Could you check a few things on this model? Use its own coordinates, in mm. Face numbers are marked on the shaded views. A direction names the side the tool comes from. Coordinates: 2 decimals unless noted, no trailing zeros. Write each loop counter-clockwise with the first axis right and the second up, starting at its lowest first coordinate (ties: lowest second). Pieces come first, ordered by that corner, then holes.
```python
from build123d import *

# Parameters (mm, degrees)
CROQUIS1_R              = 1.5
SALIENTE_EXTRUIR1_DEPTH = 10
CROQUIS2_R              = 1.5
CORTAR_EXTRUIR1_DEPTH   = 10
CROQUIS3_W              = 30
CROQUIS3_H              = 5.454139521
CORTAR_EXTRUIR2_DEPTH   = 10
REDONDEO1_R             = 5
CORTAR_EXTRUIR3_DEPTH   = 10


with BuildPart() as part:
    # Croquis1 → Saliente-Extruir1 (new body)
    with BuildSketch(Plane.XY):
        Polygon((0, 0), (15, 0), (15, 2.5), (25, 2.5), (25, 7.5), (15, 7.5), (15, 10), (0, 10), align=None)
        with Locations((5, 5)):
            Circle(CROQUIS1_R, mode=Mode.SUBTRACT)
    extrude(amount=SALIENTE_EXTRUIR1_DEPTH)

    # Croquis2 → Cortar-Extruir1 (cut)
    with BuildSketch(Plane(origin=(0, 7.5, 0), x_dir=(1, 0, 0), z_dir=(0, 1, 0))):
        with Locations(Location((20, -5, 0), (0, 0, 270))):
            Circle(CROQUIS2_R)
        with BuildLine():
            Line((20, -10), (20.922664414, -18.434540281))
            Line((20.922664414, -18.434540281), (42.481308924, -25.135304993))
            Line((42.481308924, -25.135304993), (36.797179784, -0.604681732))
            Line((36.797179784, -0.604681732), (34.226694382, 7.989532519))
            Line((34.226694382, 7.989532519), (20.461332207, 6.483723144))
            Line((20.461332207, 6.483723144), (20, 0))
            ThreePointArc((20, 0), (25, -5), (20, -10))
        make_face()
    extrude(amount=-CORTAR_EXTRUIR1_DEPTH, mode=Mode.SUBTRACT)

    # Croquis3 → Cortar-Extruir2 (cut)
    with BuildSketch(Plane(origin=(0, 10, 0), x_dir=(1, 0, 0), z_dir=(0, 1, 0))):
        with Locations((0, -10.227069761)):
            Rectangle(CROQUIS3_W, CROQUIS3_H)
        with Locations((0, 0.227069761)):
            Rectangle(CROQUIS3_W, CROQUIS3_H)
    extrude(amount=-CORTAR_EXTRUIR2_DEPTH, mode=Mode.SUBTRACT)

    # Redondeo1
    redondeo1_edges = [part.edges().sort_by_distance(p)[0] for p in [
        (0, 0, 5),
        (0, 10, 5),
    ]]
    fillet(redondeo1_edges, radius=REDONDEO1_R - 0.0001)  # a hair under: the kernel refuses the full size

    # Croquis4 → Cortar-Extruir3 (cut)
    with BuildSketch(Plane.XY.offset(7.5)):
        with BuildLine():
            Line((13.276608017, 8.188945039), (11.373430966, 10))
            Line((11.373430966, 10), (13.276608017, 11.811054961))
            ThreePointArc((13.276608017, 11.811054961), (17.5, 10), (13.276608017, 8.188945039))
        make_face()
        with BuildLine():
            Line((13.276608017, 1.811054961), (11.373430966, 0))
            Line((11.373430966, 0), (13.276608017, -1.811054961))
            ThreePointArc((13.276608017, -1.811054961), (17.5, 0), (13.276608017, 1.811054961))
        make_face()
    extrude(amount=-CORTAR_EXTRUIR3_DEPTH, mode=Mode.SUBTRACT)


solid = part.part
```
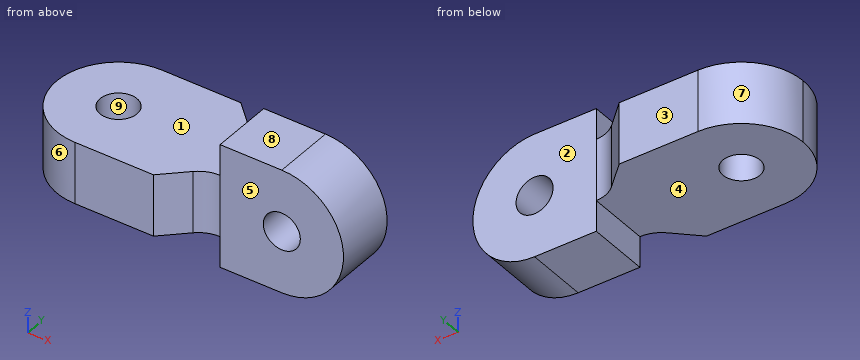
1. On a 3-axis mill with a long thin cutter (end or side, diameter ignored), from which of +Z, -Z, +X, -X, +Y, -Y can I reach the whole of each face in a straight line? I mean the marked faces 1, 2, 3, 4 and 5. Say none if no direction works.
Verdict:
face 1: +Z, -X, +Y, -Y
face 2: +Z, -Z, +X, +Y
face 3: +Z, -Z, +X, -X, +Y
face 4: -Z, -X, +Y, -Y
face 5: +Z, -Z, +X, -Y
2. I want a section at A-A on y = 4.5. Please give me the cut outline in (x, z), plus the area to 3 significant figures.
Verdict:
outline: (0.03, 2.5) - (3.59, 2.5) - (3.59, 7.5) - (0.03, 7.5) - close; (6.41, 2.5) - (15, 2.5) - (15, 0) - (20, 0) arc R5 ccw to (20, 10) - (15, 10) - (15, 7.5) - (6.41, 7.5) - close; hole circle Ø3 at (20, 5)
area: 143 mm2
3. If we mould it in two halves opening along Y, with no side actions, what happens to the marked faces 6, 7, 8 and 9? For each: pulls with the +Y half, pulls with the -Y half, needs draft (parallel to the pull), parting line crosses it, or undercut.
Verdict:
face 6: pulls with the -Y half
face 7: pulls with the +Y half
face 8: needs draft
face 9: undercut
4. For pin 1 (5 mm diameter, centred on x = 4, y = 2.5, fed in from +Z); pin 2 (1.8 mm diameter, centred on x = 5, y = 5, fed in from -Z); pin 3 (1.5 mm diameter, centred on y = 4.5, z = 2, fed in from +X); pin 4 (3 mm diameter, centred on x = 21, z = 2.5, fed in from +Y), each with a flat end and sliding along its axis, tell me the tip position at first contact or that it passes through.
Verdict:
pin 1: stops at z = 7.5
pin 2: passes through
pin 3: stops at x = 24.47
pin 4: stops at y = 7.5
5. Please list where these lines run through material, in increasing order: line 1 along Y through (x, z) = (5, 4.8); line 2 along X through (y, z) = (5, 4.4); line 3 along Z through (x, y) = (5.75, 7).
Verdict:
line 1: y = 0 to 3.5, 6.5 to 10
line 2: x = 0 to 3.5, 6.5 to 18.63, 21.37 to 24.96
line 3: z = 2.5 to 7.5
6. I want a section at C-C on y = 3. Please give me the cut outline in (x, z).
Verdict:
outline: (0.42, 2.5) - (15, 2.5) - (15, 0) - (20, 0) arc R5 ccw to (20, 10) - (15, 10) - (15, 7.5) - (0.42, 7.5) - close; hole circle Ø3 at (20, 5)
7. I want a section at D-D on z = 9. Please give me the cut outline in (x, y).
Verdict:
outline: (15, 2.5) - (23, 2.5) - (23, 7.5) - (15, 7.5) - close
8. I want a section at B-B on z = 5. Give the number of separate pieces and of enclosed holes in the cut face, plus the area to 3 significant figures.
Verdict:
separate pieces: 2
enclosed holes: 1
area: 156 mm2
